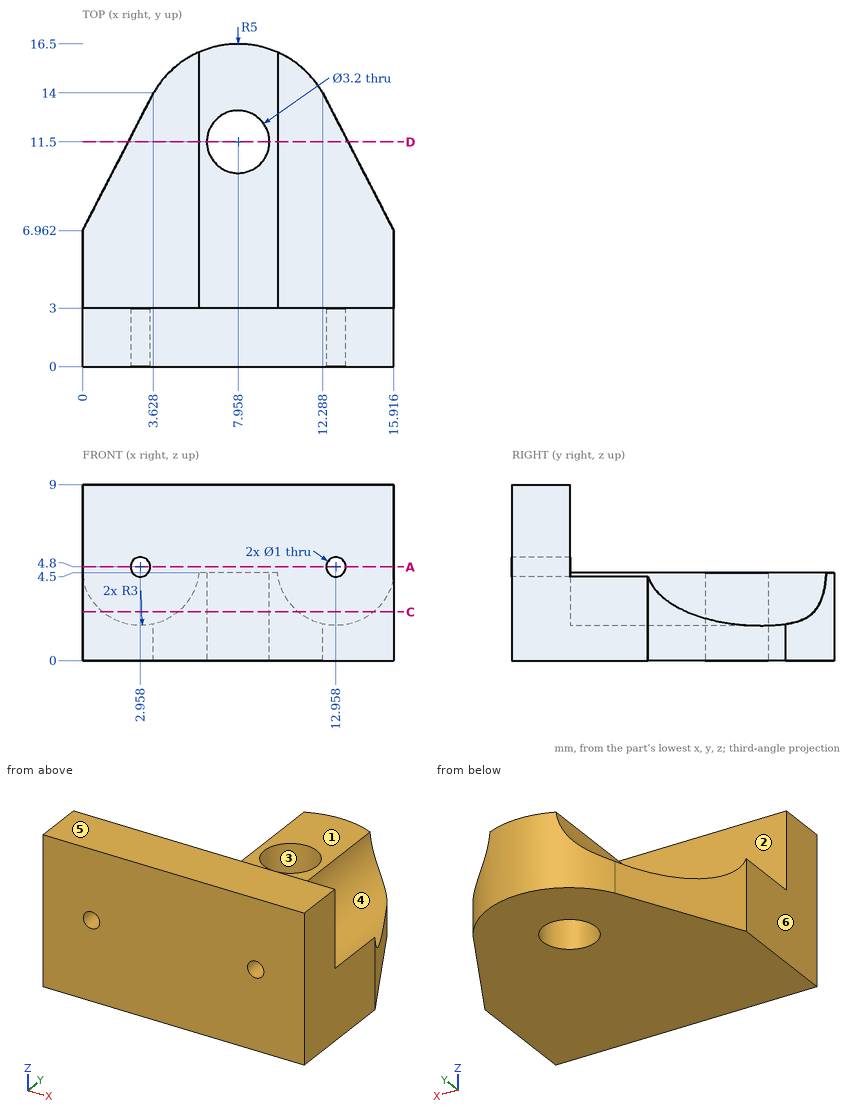
Geometry: see drawing. Coordinates: mm, zero at the bounding-box minimum. A direction names the side the tool comes from. Give positions to 0.01 mm unless a question says otherwise; leave off trailing zeros. Loops run counter-clockwise (first coordinate to the right, second up) from the corner with the lowest first, then second, coordinate; pieces in that order, holes last. Notation, with made-up numbers: (12.25, 89.5) - (26.25, 89.5) arc R17 cw to (26.25, 103.5) - close; hole circle Ø2 at (61.5, 10). An arc over 180 degrees is marked (long way). Use CSV: the item, a comma, the result in double quotes. Start each with the question number.
Item 1: Mould query, pull axis X, two halves, no side actions, for the marked faces 4, 5 and 6. Classes: pulls with the +X half, pulls with the -X half, needs draft (parallel to the pull), parting line crosses it, or undercut.
Item 2: Line query: line 1 (Y direction, x = 4.25, z = 5); line 2 (Z direction, x = 13, y = 3.5); line 3 (Y direction, x = 6.5, z = 1.5) (1 decimal). Output: solid intervals per line, ascending.
Item 3: Contact query for flat-ended pins moving along their axis: P1, Ø4, axis at x = 3, z = 4, coming from the -Y side; P2, Ø5, axis at x = 7.958, y = 11.5, coming from the +Z side; P3, Ø2, axis at x = 6.5, z = 4.5, coming from the +Y side. Output: stop coordinate, or through.
Item 4: Section A-A on z = 4.8. Return loops of the section in (x, y).
Item 5: Reachability of the marked faces 1, 2 and 3 from +Z, -Z, +X, -X, +Y, -Y: full face, straight path, thin tool, end or side. Return the list, or none.
Item 6: Section C-C on z = 2.5. Return loops of the section in (x, y) (1 decimal).
Item 7: Section D-D on y = 11.5. Return loops of the section in (x, z) (1 decimal), then the cut area to 3 significant figures.
Ans:
1,face 4,"undercut"
1,face 5,"needs draft"
1,face 6,"pulls with the -X half"
2,line 1,"y = 0 to 3"
2,line 2,"z = 0 to 1.8"
2,line 3,"y = 0 to 10.8, 12.2 to 16.3"
3,P1,"stops at y = 0"
3,P2,"stops at z = 4.5"
3,P3,"stops at y = 16.48"
4,outline,"(0, 0) - (2.46, 0) - (2.46, 3) - (0, 3) - close; (3.46, 0) - (12.46, 0) - (12.46, 3) - (3.46, 3) - close; (13.46, 0) - (15.92, 0) - (15.92, 3) - (13.46, 3) - close"
5,face 1,"+Z, +X, -X, +Y"
5,face 2,"+Z, +Y"
5,face 3,"+Z, -Z"
6,outline,"(0, 0) - (15.9, 0) - (15.9, 7) - (14.9, 9) - (14.9, 3) - (11, 3) - (11, 15.4) arc R5 ccw to (4.9, 15.4) - (4.9, 3) - (1, 3) - (1, 9) - (0, 7) - close; hole circle Ø3.2 at (8, 11.5)"
7,outline,"(2.3, 0) - (6.4, 0) - (6.4, 4.5) - (5.9, 4.5) arc R3 cw to (2.3, 1.9) - close; (9.6, 0) - (13.6, 0) - (13.6, 1.9) arc R3 cw to (10, 4.5) - (9.6, 4.5) - close"
7,area,"20.5 mm2"
